Input: part model. Units: mm. Frame: model coordinates. A direction names the side the tool comes from. Give positions to 0.01 mm unless a question says otherwise; leave off trailing zeros. Order: outer loops, then holes, each group sorted by start corner. A loop starts at its lowest first (then second) coordinate and runs counter-clockwise, first axis right, second up. Notation, with made-up numbers: (-9, 84) - (5, 84) arc R33 ccw to (5, 116) - close; hole circle Ø1 at (81.25, 13.5). An arc over 180 degrees is marked (long way). Use a Markdown table: item, result.
from build123d import *

# Parameters (mm, degrees)
SKETCH1_R                                     = 87.5
SKETCH1_R_2                                   = 82.49999999999999
BOSS_EXTRUDE1_DEPTH                           = 50
CUT_EXTRUDE1_DEPTH                            = 134.46347815039138
BOSS_EXTRUDE2_REACH                           = 201.927
BOSS_EXTRUDE2_END_RADIUS                      = 82.49999999999999
MIRROR1_AT_THE_SECOND_PLANE_COPY_1_DEPTH      = 134.46347815039138
MIRROR1_AT_THE_SECOND_PLANE_COPY_2_REACH      = 201.927
MIRROR1_AT_THE_SECOND_PLANE_COPY_2_END_RADIUS = 82.49999999999999
CUT_EXTRUDE2_DEPTH                            = 134.46347831897683
FILLET1_R                                     = 10.000000000000002


with BuildPart() as part:
    # Sketch1 → Boss-Extrude1 (new body)
    with BuildSketch(Plane.XY):
        Circle(SKETCH1_R)
        Circle(SKETCH1_R_2, mode=Mode.SUBTRACT)
    extrude(amount=BOSS_EXTRUDE1_DEPTH)

    # Sketch3 → Cut-Extrude1 (cut, through all)
    with BuildSketch(Plane(origin=(0, 0, 0), x_dir=(0, 0, 1), z_dir=(-0.7660444431189792, 0.6427876096865379, 0))):
        with BuildLine():
            Line((16, 28), (-21.31588633738815, 28))
            Line((-21.31588633738815, 28), (-21.31588633738815, -28))
            Line((-21.31588633738815, -28), (16, -28))
            ThreePointArc((16, -28), (44, 0), (16, 28))
        make_face()
    cut_extrude1 = extrude(amount=CUT_EXTRUDE1_DEPTH, mode=Mode.SUBTRACT)

    # Boss-Extrude2: up to this cylinder (the profile starts inside it)
    boss_extrude2_end = Plane(origin=(0, 0, 8), z_dir=(0, 0, -1)) * Cylinder(BOSS_EXTRUDE2_END_RADIUS, 569.8539999999999, mode=Mode.PRIVATE)
    # Sketch5 → Boss-Extrude2 (add, up to the surface)
    with BuildSketch(Plane(origin=(-53.623111018328544, 44.995132678057665, 0), x_dir=(0, 0, 1), z_dir=(-0.7660444431189792, 0.6427876096865379, 0)), mode=Mode.PRIVATE) as boss_extrude2_sk1:
        with BuildLine():
            Line((0, -28.000000000000014), (16, -28.000000000000014))
            ThreePointArc((16, -28.000000000000014), (44, -1.388e-14), (16, 27.99999999999998))
            Line((16, 27.99999999999998), (0, 27.99999999999998))
            Line((0, 27.99999999999998), (-3.7e-16, 29.99999999999998))
            Line((-3.7e-16, 29.99999999999998), (16.000000000000007, 29.999999999999982))
            ThreePointArc((16.000000000000007, 29.999999999999982), (46, -1.388e-14), (16, -30.000000000000014))
            Line((16, -30.000000000000014), (1.2e-16, -30.000000000000014))
            Line((1.2e-16, -30.000000000000014), (0, -28.000000000000014))
        make_face()
    boss_extrude2_tool1 = extrude(boss_extrude2_sk1.sketch, amount=BOSS_EXTRUDE2_REACH, mode=Mode.PRIVATE) & boss_extrude2_end
    boss_extrude2 = boss_extrude2_tool1.solids().sort_by_distance((-72.420765, 22.592961, 8))[0]
    add(boss_extrude2)

    # Mirror1: Cut-Extrude1, Boss-Extrude2 across plane
    add(cut_extrude1.mirror(Plane(origin=(0, 0, 0), x_dir=(0, 0, 1), z_dir=(1, 0, 0))), mode=Mode.SUBTRACT)
    add(boss_extrude2.mirror(Plane(origin=(0, 0, 0), x_dir=(0, 0, 1), z_dir=(1, 0, 0))))

    # Mirror1 at the second plane: Cut-Extrude1, Boss-Extrude2 across plane
    add(cut_extrude1.mirror(Plane.ZX), mode=Mode.SUBTRACT)
    add(boss_extrude2.mirror(Plane.ZX))

    # Mirror1 at the second plane copy 1 sketc → Mirror1 at the second plane copy 1 (cut, through all)
    with BuildSketch(Plane(origin=(0, 0, 0), x_dir=(0, 0, 1), z_dir=(0.7660444431189792, -0.6427876096865379, 0))):
        with BuildLine():
            Line((16, 28), (-21.31588633738815, 28))
            Line((-21.31588633738815, 28), (-21.31588633738815, -28))
            Line((-21.31588633738815, -28), (16, -28))
            ThreePointArc((16, -28), (44, 0), (16, 28))
        make_face()
    extrude(amount=MIRROR1_AT_THE_SECOND_PLANE_COPY_1_DEPTH, mode=Mode.SUBTRACT)

    # Mirror1 at the second plane copy 2: up to this cylinder (the profile starts inside it)
    mirror1_at_the_second_plane_copy_2_end = Plane(origin=(0, 0, 8), z_dir=(0, 0, -1)) * Cylinder(MIRROR1_AT_THE_SECOND_PLANE_COPY_2_END_RADIUS, 569.8539999999999, mode=Mode.PRIVATE)
    # Mirror1 at the second plane copy 2 sketc → Mirror1 at the second plane copy 2 (add, up to the surface)
    with BuildSketch(Plane(origin=(53.623111018328544, -44.995132678057665, 0), x_dir=(0, 0, 1), z_dir=(0.7660444431189792, -0.6427876096865379, 0)), mode=Mode.PRIVATE) as mirror1_at_the_second_plane_copy_2_sk1:
        with BuildLine():
            Line((0, -28.000000000000014), (16, -28.000000000000014))
            ThreePointArc((16, -28.000000000000014), (44, -1.388e-14), (16, 27.99999999999998))
            Line((16, 27.99999999999998), (0, 27.99999999999998))
            Line((0, 27.99999999999998), (-3.7e-16, 29.99999999999998))
            Line((-3.7e-16, 29.99999999999998), (16.000000000000007, 29.999999999999982))
            ThreePointArc((16.000000000000007, 29.999999999999982), (46, -1.388e-14), (16, -30.000000000000014))
            Line((16, -30.000000000000014), (1.2e-16, -30.000000000000014))
            Line((1.2e-16, -30.000000000000014), (0, -28.000000000000014))
        make_face()
    mirror1_at_the_second_plane_copy_2_tool1 = extrude(mirror1_at_the_second_plane_copy_2_sk1.sketch, amount=MIRROR1_AT_THE_SECOND_PLANE_COPY_2_REACH, mode=Mode.PRIVATE) & mirror1_at_the_second_plane_copy_2_end
    add(mirror1_at_the_second_plane_copy_2_tool1.solids().sort_by_distance((-72.420765, 22.592961, 8))[0])

    # Sketch4 → Cut-Extrude2 (cut, through all)
    with BuildSketch(Plane.XY.offset(50)):
        Polygon((-37.5, 150.50625054825755), (37.5, 150.50625054825755), (37.49999999999998, 0), (-37.49999999999998, 0), align=None)
    extrude(amount=-CUT_EXTRUDE2_DEPTH, mode=Mode.SUBTRACT)

    # Fillet1
    fillet1_edges = [part.edges().sort_by_distance(p)[0] for p in [
        (37.49999999999999, 76.2708168938525, 50),
        (-37.49999999999999, 76.2708168938529, 50),
    ]]
    fillet(fillet1_edges, radius=FILLET1_R)


solid = part.part
1. Material intervals for line 1 along X through (y, z) = (0, 14); line 2 along Y through (x, z) = (0, 16.5); line 3 along Y through (x, z) = (43, 35.5), sorted ascending.
Response:
| item | result |
|---|---|
| line 1 | x = -87.5 to -82.5, 82.5 to 87.5 |
| line 2 | y = -87.5 to -82.5 |
| line 3 | y = -76.21 to -70.41, -65.84 to -62.31, 62.31 to 65.84, 70.41 to 76.21 |
2. Set-up query: faces 4 (the face through (40.497, -70.532, 8.112)), 5 (the face through (75.495, -24.185, 8.112)), 6 (the face through (-40.497, -70.532, 8.112)). Return all of +Z, -Z, +X, -X, +Y, -Y with unobstructed straight access to the full face (end or side cutting, diameter ignored); none if empty.
Response:
| item | result |
|---|---|
| face 4 | -Z, +X |
| face 5 | +Z, -Z |
| face 6 | -Z, -X |
3. Section query C-C (x = 0). Return loops of the section in (y, z).
Response:
| item | result |
|---|---|
| outline | (-87.5, 0) - (-82.5, 0) - (-82.5, 50) - (-87.5, 50) - close |
4. Section query A-A (y = 0). Return loops of the section in (x, z), then the cut area to 3 significant figures.
Response:
| item | result |
|---|---|
| outline | (-87.5, 0) - (-82.5, 0) - (-82.5, 50) - (-87.5, 50) - close; (82.5, 0) - (87.5, 0) - (87.5, 50) - (82.5, 50) - close |
| area | 500 mm^2 |
5. Pin query (flat end, axial travel): pin 1 (1.9 mm diameter, centred on y = 68, z = 12.5, fed in from -X); pin 2 (4 mm diameter, centred on y = -8, z = 21.5, fed in from -X); pin 3 (1 mm diameter, centred on y = 62, z = 43.5, fed in from +X). Return the tip coordinate at first contact, or that it passes through.
Response:
| item | result |
|---|---|
| pin 1 | stops at x = -38.61 |
| pin 2 | stops at x = -87.29 |
| pin 3 | stops at x = 62.24 |
6. Section query B-B (z = 10). State how many separate pieces and enclosed holes the cut face has, then the cut area to 3 significant figures.
Response:
| item | result |
|---|---|
| separate pieces | 5 |
| enclosed holes | 0 |
| area | 1,240 mm^2 |
7. Mould query, pull axis Y, two halves, no side actions, for faces 1 (the face through (-3.305, -87.438, 30.206)), 2 (the face through (59.148, -48.827, 43.993)), 3 (the face through (37.5, 76, 20)). Classes: pulls with the +Y half, pulls with the -Y half, needs draft (parallel to the pull), parting line crosses it, or undercut.
Response:
| item | result |
|---|---|
| face 1 | parting line crosses it |
| face 2 | undercut |
| face 3 | needs draft |
